```python
from build123d import *

# Parameters (mm, degrees)
F2_R     = 122
F2_R_2   = 102
F3_DEPTH = 5
F4_R     = 32
F4_R_2   = 12
F5_DEPTH = 5
F6_R     = 5
F7_DEPTH = 425.8855726812
F8_R     = 5
F9_DEPTH = 5


with BuildPart() as f1:
    # F0 (on Front) → F1 (revolve)
    with BuildSketch(Plane.XZ):
        Polygon((-100, 195.8845726812), (-100, 425.8845726812), (-102, 425.8845726812), (-102, 195.3486742963), (-12, 39.4641016151), (-12, 0), (-10, 0), (-10, 40), align=None)
    revolve(axis=Axis((0, 0, 212.9422863406), (0, 0, 1)))

    # F2 (on face) → F3 (join)
    with BuildSketch(Plane.XY.offset(425.8845726812)):
        Circle(F2_R)
        Circle(F2_R_2, mode=Mode.SUBTRACT)
    extrude(amount=-F3_DEPTH)

    # F4 (on face) → F5 (join)
    with BuildSketch(Plane(origin=(0, 0, 0), x_dir=(1, 0, 0), z_dir=(0, 0, -1))):
        Circle(F4_R)
        Circle(F4_R_2, mode=Mode.SUBTRACT)
    extrude(amount=-F5_DEPTH)

    # F6 (on face) → F7 (cut, through all)
    with BuildSketch(Plane.XY.offset(425.8845726812)):
        with Locations((0, 110)):
            Circle(F6_R)
        with Locations((-95.2627944163, 55)):
            Circle(F6_R)
        with Locations((-95.2627944163, -55)):
            Circle(F6_R)
        with Locations((0, -110)):
            Circle(F6_R)
        with Locations((95.2627944163, -55)):
            Circle(F6_R)
        with Locations((95.2627944163, 55)):
            Circle(F6_R)
    extrude(amount=-F7_DEPTH, mode=Mode.SUBTRACT)

    # F8 (on face) → F9 (cut, through all)
    with BuildSketch(Plane(origin=(0, 0, 0), x_dir=(1, 0, 0), z_dir=(0, 0, -1))):
        with Locations((0, 20)):
            Circle(F8_R)
        with Locations((-20, 0)):
            Circle(F8_R)
        with Locations((0, -20)):
            Circle(F8_R)
        with Locations((20, 0)):
            Circle(F8_R)
    extrude(amount=-F9_DEPTH, mode=Mode.SUBTRACT)


solid = f1.part
```
Geometry check sheet. Reference: the model listing, model coordinates, mm. A direction names the side the tool comes from. Coordinates: 2 decimals unless noted, no trailing zeros. Write each loop counter-clockwise with the first axis right and the second up, starting at its lowest first coordinate (ties: lowest second). Pieces come first, ordered by that corner, then holes. Notation, with made-up numbers: M -28,47.25 L -20,47.25 A22 cw -20,81.25 Z; hole C 8,-1.5 d9. An arc over 180 degrees is marked long. Use one line per item in the form item = value. Start each with the question number.
1) Thickness scan on probe 1 along X at (y, z) = (0, 3); probe 2 along Y at (x, z) = (0, 422.3). Record the ranges inside material, lowest first. Write a range as from..to.
2) Section check A-A on y = 0. State how many separate pieces and enclosed holes the cut face has, and give its area (3 significant figures).
3) Release check for a two-part mould opening along X. For faces 1 (the cylindrical face through (-25, 0, 2)), 2 (the cylindrical face through (22.112, 99.574, 306.538)), 3 (the flat face through (7, -8, 0)) record: pulls with the +X half, pulls with the -X half, needs draft (parallel to the pull), parting line crosses it, or undercut.
4) Section check B-B on z = 378. Enter the section's corners in (x, y), and give its area (3 significant figures).
5) Set-up check for faces 4 (the cylindrical face through (-95.38, -30.04, 312.49)), 5 (the cylindrical face through (-92.575, -50.784, 423.42)), 6 (the cylindrical face through (15, 0, 2)), 7 (the flat face through (14, 0, 5)): record each of +Z, -Z, +X, -X, +Y, -Y from which the full face is reachable in a straight line by a thin tool's end or side.
6) Go/stop test with flat-tipped pins: pin 1 Ø9 at (x, y) = (0, 110) entering from -Z; pin 2 Ø1 at (x, y) = (67.5, -19.5) entering from -Z; pin 3 Ø11.5 at (x, y) = (-20, 0) entering from +Z; pin 4 Ø1.5 at (x, y) = (48, 34) entering from -Z. Record where each tip stops, or that it passes through.
Responses:
q1.probe_1 = -32..-25, -15..-10, 10..15, 25..32
q1.probe_2 = -122..-115, -105..-100, 100..105, 115..122
q2.separate_pieces = 4
q2.enclosed_holes = 0
q2.area = 2,100 mm2
q3.face_1 = undercut
q3.face_2 = parting line crosses it
q3.face_3 = needs draft
q4.outline = C 0,0 d204; hole C 0,0 d200
q4.area = 1,270 mm2
q5.face_4 = +Z
q5.face_5 = +Z, -Z
q5.face_6 = -Z
q5.face_7 = none
q6.pin_1 = through
q6.pin_2 = 139.51
q6.pin_3 = 67.28
q6.pin_4 = 119.26
